The listing builds one solid part. Answer for the finished solid, in the listing's coordinates (mm). Face numbers are marked on the shaded views. A direction names the side the tool comes from. Coordinates: 2 decimals unless noted, no trailing zeros. Order: outer loops, then holes, each group sorted by start corner. A loop starts at its lowest first (then second) coordinate and runs counter-clockwise, first axis right, second up.
from build123d import *

# Parameters (mm, degrees)
F0_W      = 609.6
F0_H      = 304.8
F1_DEPTH  = 19.05
F2_W      = 533.4
F2_H      = 228.6
F3_DEPTH  = 19.05
F4_R      = 42.8625
F5_DEPTH  = 6.35
F6_R      = 12.7
F7_DEPTH  = 215.9
F8_R      = 42.8625
F9_DEPTH  = 6.35
F10_W     = 88.9
F10_H     = 88.9
F11_DEPTH = 38.1
F12_SIZE  = 63.5


with BuildPart() as f1:
    # F0 (on Top) → F1 (new body)
    with BuildSketch(Plane.XY):
        Rectangle(F0_W, F0_H)
    extrude(amount=F1_DEPTH)

    # F2 (on face) → F3 (join)
    with BuildSketch(Plane.XY.offset(19.05)):
        Rectangle(F2_W, F2_H)
    extrude(amount=F3_DEPTH)

    # F4 (on face) → F5 (join)
    with BuildSketch(Plane.XY.offset(38.1)):
        with Locations((-190.5, 0)):
            Circle(F4_R)
        with Locations((190.5, 0)):
            Circle(F4_R)
    extrude(amount=F5_DEPTH)

    # F6 (on face) → F7 (join)
    with BuildSketch(Plane.XY.offset(44.45)):
        with Locations((-190.5, 0)):
            Circle(F6_R)
        with Locations((190.5, 0)):
            Circle(F6_R)
    extrude(amount=F7_DEPTH)

    # F8 (on face) → F9 (join)
    with BuildSketch(Plane.XY.offset(260.35)):
        with Locations((-190.5, 0)):
            Circle(F8_R)
        with Locations((190.5, 0)):
            Circle(F8_R)
    extrude(amount=F9_DEPTH)

    # F10 (on face) → F11 (join)
    with BuildSketch(Plane.XY.offset(266.7)):
        with Locations((-190.5, 0)):
            Rectangle(F10_W, F10_H)
        with Locations((190.5, 0)):
            Rectangle(F10_W, F10_H)
    extrude(amount=F11_DEPTH)

    # F12
    f12_edges = [f1.edges().sort_by_distance(p)[0] for p in [
        (-266.7, 114.3, 28.575),
        (-266.7, -114.3, 28.575),
        (-304.8, -152.4, 9.525),
        (-304.8, 152.4, 9.525),
        (266.7, 114.3, 28.575),
        (266.7, -114.3, 28.575),
        (304.8, 152.4, 9.525),
        (304.8, -152.4, 9.525),
    ]]
    chamfer(f12_edges, length=F12_SIZE)


solid = f1.part
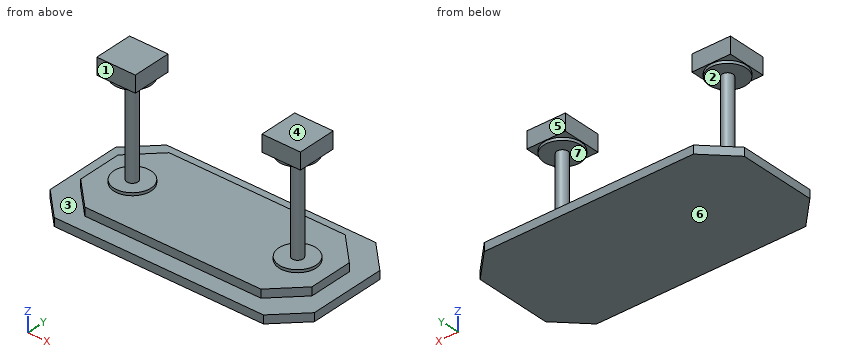
(1) Given pin 1 Ø1.5 at (x, y) = (-128.5, 73) entering from +Z; pin 2 Ø21 at (x, z) = (-62, 32) entering from -Y; pin 3 Ø12 at (y, z) = (-7, 158) entering from +X; pin 4 Ø21 at (y, z) = (-17, 27.5) entering from +X, each flat-ended and moving along its own axis, determine where each tip first touches the part or whether it passes through.
(2) Find the intervals of material crossed by probe 1 along Z at (x, y) = (-162, -28); probe 2 along Z at (x, y) = (168.5, 37); probe 3 along Z at (x, y) = (30, 110), in increasing order.
(3) Find section D-D on x = -190.5. Determine the outline of the cut face in (y, z).
(4) The mould has two halves that part along Z. Classify the marked faces 4, 5, 6 and 7: pulls with the +Z half, pulls with the -Z half, needs draft (parallel to the pull), parting line crosses it, or undercut.
(5) A tool of negligible diameter and unlimited length cuts with its end or side. For the marked faces 1, 2 and 3, from which of +Z, -Z, +X, -X, +Y, -Y can it reach the whole face along a straight path? Write none if from no direction.
(6) Find section C-C on z = 196. Determine the outline of the cut face in (x, y).
(7) Find section B-B on y = -82.5. Determine the outline of the cut face in (x, z).
(8) Find section A-A on x = 86.5. Determine the outline of the cut face in (y, z).
Resolved:
1. pin 1: stops at z = 38.1
1. pin 2: stops at y = -114.3
1. pin 3: stops at x = 203.16
1. pin 4: stops at x = 304.8
2. probe 1: z = 0 to 44.45, 260.35 to 304.8
2. probe 2: z = 0 to 38.1, 266.7 to 304.8
2. probe 3: z = 0 to 38.1
3. outline: (-152.4, 0) - (152.4, 0) - (152.4, 19.05) - (114.3, 19.05) - (114.3, 38.1) - (42.86, 38.1) - (42.86, 44.45) - (12.7, 44.45) - (12.7, 260.35) - (42.86, 260.35) - (42.86, 266.7) - (44.45, 266.7) - (44.45, 304.8) - (-44.45, 304.8) - (-44.45, 266.7) - (-42.86, 266.7) - (-42.86, 260.35) - (-12.7, 260.35) - (-12.7, 44.45) - (-42.86, 44.45) - (-42.86, 38.1) - (-114.3, 38.1) - (-114.3, 19.05) - (-152.4, 19.05) - close
4. face 4: pulls with the +Z half
4. face 5: needs draft
4. face 6: pulls with the -Z half
4. face 7: undercut
5. face 1: +Z, +X, -X, -Y
5. face 2: none
5. face 3: +Z
6. outline: circle Ø25.4 at (-190.5, 0); circle Ø25.4 at (190.5, 0)
7. outline: (-304.8, 0) - (304.8, 0) - (304.8, 19.05) - (235, 19.05) - (235, 38.1) - (-235, 38.1) - (-235, 19.05) - (-304.8, 19.05) - close
8. outline: (-152.4, 0) - (152.4, 0) - (152.4, 19.05) - (114.3, 19.05) - (114.3, 38.1) - (-114.3, 38.1) - (-114.3, 19.05) - (-152.4, 19.05) - close
